Autodesk Inventor part; units mm, degrees
ref_plane "YZ Plane" through (0, 0, 0) normal (1, 0, 0) x (0, 1, 0)
ref_plane "XZ Plane" through (0, 0, 0) normal (0, 1, 0) x (-1, 0, 0)
ref_plane "XY Plane" through (0, 0, 0) normal (0, 0, 1) x (1, 0, 0)
sketch "Sketch1" plane through (0, 0, 0) normal (0, 1, 0) x (-1, 0, 0)
  line L0 (54.5284, -163.8048) -> (49.6951, -172.1764)
  arc A0 (49.6951, -172.1764) -> (50.8498, -174.1764) centre (50.8498, -172.843) ccw
  line L1 (50.8498, -174.1764) -> (117.5164, -174.1764)
  line L2 (113.8378, -163.8048) -> (118.6711, -172.1764)
  arc A1 (117.5164, -174.1764) -> (118.6711, -172.1764) centre (117.5164, -172.843) ccw
  arc A2 (259.3338, -380.9628) -> (202.7682, -171.3935) centre (-165.66, -383.2559) ccw
  line L3 (113.8378, -163.8048) -> (118.3961, -163.8048)
  arc A3 (118.3961, -163.8048) -> (118.4865, -161.1412) centre (118.3961, -162.4715) ccw
  line L4 (54.5284, -163.8048) -> (49.9178, -163.8048)
  arc A4 (49.9178, -161.1381) -> (49.9178, -163.8048) centre (49.9178, -162.4715) ccw
  line L5 (5.6828, -148.1362) -> (5.6828, -142.6365)
  line L6 (5.6828, -142.6365) -> (11.6828, -142.6364)
  line L7 (11.6828, -142.6364) -> (11.6828, -145.4697)
  arc A5 (11.6828, -145.4697) -> (11.6828, -148.1364) centre (11.6828, -146.803) ccw
  arc A6 (3.0183, -148.0602) -> (5.6828, -148.1362) centre (4.3494, -148.1362) ccw
  line L8 (162.7021, -148.1362) -> (162.7021, -142.6363)
  line L9 (162.7021, -142.6363) -> (156.7021, -142.6363)
  line L10 (156.7021, -142.6363) -> (156.7021, -145.4697)
  arc A7 (156.7021, -148.1364) -> (156.7021, -145.4697) centre (156.7021, -146.803) ccw
  arc A8 (162.7021, -148.1362) -> (165.3666, -148.0602) centre (164.0355, -148.1362) ccw
  line L11 (165.3666, -148.0602) -> (179.8476, -148.0602)
  line L12 (179.8476, -148.0602) -> (179.8476, -168.7268)
  arc A9 (179.8476, -168.7268) -> (179.8476, -171.3935) centre (179.8476, -170.0602) ccw
  line L13 (179.8476, -171.3935) -> (202.7682, -171.3935)
  line L14 (78.171, -370.9703) -> (69.785, -370.9703)
  line L15 (168.6888, -389.73) -> (168.6888, -432.7538)
  arc A10 (201.1888, -413.0028) -> (202.3435, -411.0028) centre (201.1888, -411.6694) ccw
  line L16 (195.5003, -397.8103) -> (195.5003, -373.6294)
  arc A11 (195.5003, -370.9628) -> (195.5003, -373.6294) centre (195.5003, -372.2961) ccw
  line L17 (195.5003, -370.9628) -> (202.0003, -370.9628)
  arc A12 (202.0003, -373.6294) -> (202.0003, -370.9628) centre (202.0003, -372.2961) ccw
  line L18 (202.0003, -373.6294) -> (202.0003, -380.9628)
  line L19 (78.1632, -380.9628) -> (135.4967, -380.9628)
  line L20 (202.0003, -380.9628) -> (259.3338, -380.9628)
  arc A13 (135.0341, -411.0028) -> (136.1888, -413.0028) centre (136.1888, -411.6694) ccw
  arc A14 (141.8773, -373.6233) -> (142.0056, -370.9628) centre (142.0056, -372.2961) ccw
  line L21 (142.0056, -370.9628) -> (135.5056, -370.9628)
  arc A15 (135.5056, -370.9628) -> (135.5032, -373.6294) centre (135.5056, -372.2961) ccw
  line L22 (135.5032, -373.6294) -> (135.4967, -380.9628)
  line L23 (49.9178, -161.1381) -> (49.9178, -148.1364)
  line L24 (118.4865, -148.1364) -> (118.4865, -161.1412)
  line L25 (202.3435, -411.0028) -> (196.1702, -400.3103)
  arc A16 (195.5003, -397.8103) -> (196.1702, -400.3103) centre (200.5003, -397.8103) ccw
  line L26 (141.8773, -397.8103) -> (141.8773, -373.6233)
  line L27 (135.0341, -411.0028) -> (141.2075, -400.3103)
  arc A17 (141.2075, -400.3103) -> (141.8773, -397.8103) centre (136.8773, -397.8103) ccw
  arc A18 (78.1697, -373.637) -> (78.171, -370.9703) centre (78.171, -372.3036) ccw
  line L28 (78.1632, -380.9628) -> (78.1697, -373.637)
  line L29 (136.1888, -413.0028) -> (201.1888, -413.0028)
  arc A19 (-9.9624, -148.0602) -> (-11.0329, -150.3848) centre (-9.9624, -149.469) ccw
  arc A20 (69.785, -370.9703) -> (-10.5152, -151.1127) centre (-579.254, -483.4304) ccw
  arc A21 (-10.5152, -151.1127) -> (-11.0329, -150.3848) centre (-14.8322, -153.6352) ccw
  line L30 (118.4865, -148.1364) -> (156.7021, -148.1364)
  line L31 (84.1831, -174.1764) -> (84.1831, -204.8832)
  line L32 (-9.9624, -148.0602) -> (3.0183, -148.0602)
  line L33 (11.6828, -148.1364) -> (49.9178, -148.1364)
  point P0 (2.7021, -144.053)
  point P1 (1.3688, -146.803)
  point P2 (-3.2979, -145.3864)
  point P3 (-7.9624, -148.0602)
  point P4 (116.117, -163.8048)
  dimension "d102" = 2.6667
  dimension "d107" = 2.6667
  dimension "d108" = 6.5
  dimension "d109" = 2.6667
  dimension "d111" = 57.3335
  dimension "d127" = 9.6667
  dimension "d128" = 9.6667
  dimension "d129" = 1.3333
  dimension "d131" = 62.3312
  dimension "d132" = 1.3333
  dimension "d133" = 14.481
  dimension "d134" = 1.3333
  dimension "d135" = 6
  dimension "d141" = 7.3333
  dimension "d142" = 5
  dimension "d145" = 1.3333
  dimension "d149" = 1.3333
  dimension "d151" = 658.71
  dimension "d152" = 5
  dimension "d153" = 68.5687
  dimension "d154" = 66.6667
  dimension "d155" = 1.3333
  dimension "d156" = 1.3333
  dimension "d158" = 1.3333
  dimension "d160" = 10.3716
  dimension "d161" = 10.3716
  dimension "d162" = 38.2156
  dimension "d163" = 38.235
  dimension "d164" = 15.6684
  dimension "d165" = 15.6684
  dimension "d166" = 23.3333
  dimension "d167" = 84.5058
  dimension "d169" = 264.8664
  dimension "d170" = 145.0381
  dimension "d171" = 6
  dimension "d172" = 5.4997
  dimension "d173" = 1.3333
  dimension "d174" = 2.8333
  dimension "d175" = 145.0006
extrude "Extrusion3" add sketch "Sketch1" along normal blind 6
properties part number "Support B"
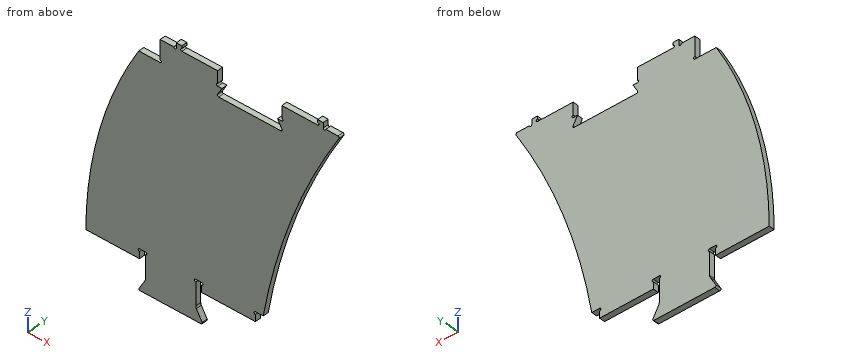
Source: CAD feature listing. Evaluate the final solid. Frame: model axes, mm. Round coordinates to 2 decimals unless told otherwise and drop trailing zeros. Order: outer loops, then holes, each group sorted by start corner. A loop starts at its lowest first (then second) coordinate and runs counter-clockwise, first axis right, second up. Notation, with made-up numbers: (13.25, 38) - (47.25, 38) arc R27 ccw to (47.25, 70) - close; hole circle Ø6 at (-8, 37.25). An arc over 180 degrees is marked (long way). Use a Markdown table: item, result. Add a question column.
1. First-contact query: pin 1 (1.4 mm diameter, centred on x = -115, y = 2, fed in from +Z); pin 2 (2.5 mm diameter, centred on y = 2.5, z = -146.5, fed in from -X); pin 3 (1.5 mm diameter, centred on x = -193.5, y = 5, fed in from +Z). Flat tips, straight axial feed; report the tip coordinate or a pass-through.
2. Section query B-B (x = -84). Return the cut outline in (y, z).
3. Line query: probe 1 along Z at (x, y) = (-124, 1.35); probe 2 along Z at (x, y) = (-176, 5.45); probe 3 along X at (y, z) = (4.4, -393). Output: solid intervals per line, ascending.
4. Section query A-A (z = -393). Return the cut outline in (x, y), then the cut area to 3 significant figures.
Derived:
| question | item | result |
|---|---|---|
| 1 | pin 1 | z = -163.8 |
| 1 | pin 2 | x = -162.7 |
| 1 | pin 3 | z = -171.39 |
| 2 | outline | (0, -380.96) - (6, -380.96) - (6, -174.18) - (0, -174.18) - close |
| 3 | probe 1 | -380.96 to -148.14 |
| 3 | probe 2 | -413 to -148.06 |
| 3 | probe 3 | -195.5 to -141.88 |
| 4 | outline | (-195.5, 0) - (-141.88, 0) - (-141.88, 6) - (-195.5, 6) - close |
| 4 | area | 322 mm2 |
